Could you check a few things on this model? Use its own coordinates, in mm. A direction names the side the tool comes from. Give positions to 0.01 mm unless a question says otherwise; leave off trailing zeros. Loops run counter-clockwise (first coordinate to the right, second up) from the corner with the lowest first, then second, coordinate; pieces in that order, holes last. Notation, with made-up numbers: M -35,12.5 L -30,12.5 A17 cw -30,37.5 Z; hole C -17.5,3 d7. An arc over 180 degrees is marked long. Use a Markdown table: item, result. Add a question column.
1) Suppose I cut it at D-D on y = 71. List the corners of the cut face in (x, z) for me, and give its area (3 significant figures).
2) If I drill on line 1 along Y through (x, z) = (2.5, -18.5); line 2 along X through (y, z) = (62, 0); line 3 along Z through (x, y) = (0, 62.5), over which ranges is the centre line in solid material (lowest first)? Write a range as [from, to].
3) Will these pins go through, and if not, where does the flat tip stop? pin 1 Ø4 at (y, z) = (63, -25.5) entering from -X; pin 2 Ø17.5 at (y, z) = (44.5, -14.5) entering from -X; pin 3 Ø10 at (x, z) = (-4.5, -27) entering from +Y.
4) We'd pull the mould along Y, two halves only. Please class faces 6 (the flat face through (6, 65, -23)), 7 (the cylindrical face through (1.14, 31.85, 19.25)), 8 (the flat face through (0, 0, -9)), 9 (the flat face through (-13, 50, 0)): +Y half, -Y half, draft (parallel to the pull), parting line (faces both ways), or undercut.
5) Suppose I cut it at C-C on z = 0. List the corners of the cut face in (x, y) for me.
6) Suppose I cut it at B-B on y = 34.5. List the corners of the cut face in (x, z) for me, and give its area (3 significant figures).
7) Suppose I cut it at A-A on z = -16.5. List the corners of the cut face in (x, y) for me.
8) Which directions (+Z, -Z, +X, -X, +Y, -Y) give clear straight access to the entire face, cutting with the end or side of a thin tool? Please do faces 1 (the cylindrical face through (5, 65, -34)), 2 (the flat face through (11.774, 62.762, 8.74)), 3 (the flat face through (-1, 80, 13)), 4 (the cylindrical face through (-7.835, 64.345, 9.739)), 5 (the cylindrical face through (0.15, 48.33, 13.25)).
```python
from build123d import *
from OCP.BRepFilletAPI import BRepFilletAPI_MakeFillet

# Parameters (mm, degrees)
SKETCH1_R               = 12.5
BOSS_EXTRUDE1_DEPTH     = 80
CUT_EXTRUDE1_DEPTH      = 88.77439656
CUT_EXTRUDE1_DEPTH_BACK = 88.77439656
SKETCH4_OUTSIDE_W       = 61.818
SKETCH4_OUTSIDE_H       = 100.83
SKETCH6_W               = 20
SKETCH6_H               = 8.19180338
SKETCH6_W_2             = 12
SKETCH6_H_2             = 19
BOSS_EXTRUDE3_DEPTH     = 50
CUT_EXTRUDE2_START      = -30
SKETCH8_R               = 12.5
CUT_EXTRUDE2_DEPTH      = 30
FILLET1_R               = 5
FILLET2_R               = 15
FILLET3_R1              = 1
FILLET3_R2              = 5
CUT_EXTRUDE4_DEPTH      = 84.91706908
CUT_EXTRUDE4_DEPTH_BACK = 84.91706908
SKETCH11_R              = 1.55
FILLET4_R               = 10
SKETCH12_R              = 5.25
CUT_EXTRUDE5_DEPTH      = 96.372952239


with BuildPart() as part:
    # Sketch1 → Boss-Extrude1 (new body)
    with BuildSketch(Plane(origin=(0, 0, 0), x_dir=(1, 0, 0), z_dir=(0, 1, 0))):
        with BuildLine():
            Line((-13.243243243, -4.540540541), (-10, -14))
            Line((-10, -14), (-10, -26.98786193))
            Line((-10, -26.98786193), (10, -26.98786193))
            Line((10, -26.98786193), (10, -14))
            Line((10, -14), (13.597983435, -3.330892747))
            ThreePointArc((13.597983435, -3.330892747), (-0.630295246, 13.985804514), (-13.243243243, -4.540540541))
        make_face()
        with Locations(Location((0, 0, 0), (0, 0, 270))):
            Circle(SKETCH1_R, mode=Mode.SUBTRACT)
    extrude(amount=BOSS_EXTRUDE1_DEPTH)

    # Sketch4 outside → Cut-Extrude1 (cut, two sides: drawn at the far end of the back side and taken through both)
    with BuildSketch(Plane.ZY.offset(10).offset(-CUT_EXTRUDE1_DEPTH_BACK)):
        with Locations((6.494, 40)):
            Rectangle(SKETCH4_OUTSIDE_W, SKETCH4_OUTSIDE_H)
        with BuildLine():
            Line((-10, 50), (10, 50))
            ThreePointArc((10, 50), (12.828427125, 48.828427125), (14, 46))
            Line((14, 46), (14, 0))
            Line((14, 0), (23.289589956, 0))
            ThreePointArc((23.289589956, 0), (26.209542913, 8.210116535), (25.999737715, 16.921495334))
            Line((25.999737715, 16.921495334), (19.944041303, 78.646458452))
            ThreePointArc((19.944041303, 78.646458452), (19.458758034, 79.611235276), (18.451208451, 80))
            Line((18.451208451, 80), (14, 80))
            Line((14, 80), (-10, 80))
            ThreePointArc((-10, 80), (-12.828427125, 78.828427125), (-14, 76))
            Line((-14, 76), (-14, 54))
            ThreePointArc((-14, 54), (-12.828427125, 51.171572875), (-10, 50))
        make_face(mode=Mode.SUBTRACT)
    extrude(amount=CUT_EXTRUDE1_DEPTH + CUT_EXTRUDE1_DEPTH_BACK, mode=Mode.SUBTRACT)

    # Sketch6 → Boss-Extrude3 (add)
    with BuildSketch(Plane(origin=(0, 0, 14), x_dir=(-1, 0, 0), z_dir=(0, 0, -1))):
        with Locations((0, 4.09590169)):
            Rectangle(SKETCH6_W, SKETCH6_H)
        with Locations((0, 64.998822006)):
            Rectangle(SKETCH6_W_2, SKETCH6_H_2)
    extrude(amount=BOSS_EXTRUDE3_DEPTH)

    # Sketch8 → Cut-Extrude2 (cut)
    with BuildSketch(Plane(origin=(0, 80, 0), x_dir=(1, 0, 0), z_dir=(0, 1, 0)).offset(CUT_EXTRUDE2_START)):
        with Locations(Location((0, 0, 0), (0, 0, 53.130102354))):
            Circle(SKETCH8_R)
    extrude(amount=CUT_EXTRUDE2_DEPTH, mode=Mode.SUBTRACT)

    # Fillet1
    fillet1_edges = [part.edges().sort_by_distance(p)[0] for p in [
        (10, 4.09590169, -36),
        (-10, 4.09590169, -36),
        (6, 64.998822006, -36),
        (-6, 64.998822006, -36),
    ]]
    fillet(fillet1_edges, radius=FILLET1_R)

    # Fillet2
    fillet2_edges = [part.edges().sort_by_distance(p)[0] for p in [
        (0, 8.19180338, 14),
    ]]
    fillet(fillet2_edges, radius=FILLET2_R)

    # Fillet3: one fillet with a radius per group of edges: ONE call of the kernel's fillet builder (fillet() takes one radius for all edges)
    fillet3_edges_1 = [part.edges().sort_by_distance(p)[0] for p in [
        (0, 74.498822006, -14),
        (0, 55.498822006, -14),
    ]]
    fillet3_edges_2 = [part.edges().sort_by_distance(p)[0] for p in [
        (-6, 64.998822006, -12.649110641),
        (6, 64.998822006, -12.649110641),
    ]]
    fillet3 = BRepFilletAPI_MakeFillet(part.part.solid().wrapped)
    for e in fillet3_edges_1:
        fillet3.Add(FILLET3_R1, e.wrapped)
    for e in fillet3_edges_2:
        fillet3.Add(FILLET3_R2, e.wrapped)
    add(Compound.cast(fillet3.Shape()), mode=Mode.REPLACE)

    # Sketch11 → Cut-Extrude4 (cut, two sides: drawn at the far end of the back side and taken through both)
    with BuildSketch(Plane(origin=(0, 74.498822006, 0), x_dir=(1, 0, 0), z_dir=(0, 1, 0)).offset(-CUT_EXTRUDE4_DEPTH_BACK)):
        with Locations(Location((0, 31.585251235, 0), (0, 0, 270))):
            Circle(SKETCH11_R)
    extrude(amount=CUT_EXTRUDE4_DEPTH + CUT_EXTRUDE4_DEPTH_BACK, mode=Mode.SUBTRACT)

    # Fillet4
    fillet4_edges = [part.edges().sort_by_distance(p)[0] for p in [
        (0, 16.921495334, 25.999737715),
        (0, 0, 23.289589956),
    ]]
    fillet(fillet4_edges, radius=FILLET4_R)

    # Sketch12 → Cut-Extrude5 (cut, through all)
    with BuildSketch(Plane(origin=(0, 0, 14), x_dir=(-1, 0, 0), z_dir=(0, 0, -1))):
        with Locations((0, 36.973808643)):
            Circle(SKETCH12_R)
    extrude(amount=-CUT_EXTRUDE5_DEPTH, mode=Mode.SUBTRACT)


solid = part.part
```
Answer block:
| question | item | result |
|---|---|---|
| 1 | outline | M -13.24,4.54 A14 ccw -8.11,-11.42 A5 cw -6,-15.49 L -6,-31 A5 ccw -1,-36 L 1,-36 A5 ccw 6,-31 L 6,-15.49 A5 cw 8.11,-11.42 A14 ccw 13.6,3.33 L 10,14 L 10,20.69 L -10,20.69 L -10,14 Z; hole C 0,0 d25; hole C 0,-31.59 d3.1 |
| 1 | area | 549 mm^2 |
| 2 | line 1 | y = [0, 8.19], [55.5, 74.5] |
| 2 | line 2 | x = [-14, -12.5], [12.5, 14] |
| 2 | line 3 | z = [-36, -33.14], [-30.04, -12.5], [12.5, 21.53] |
| 3 | pin 1 | stops at x = -6 |
| 3 | pin 2 | stops at x = -11.7 |
| 3 | pin 3 | stops at y = 74.5 |
| 4 | face 6 | draft |
| 4 | face 7 | undercut |
| 4 | face 8 | -Y half |
| 4 | face 9 | undercut |
| 5 | outline | M -14,50 L -12.5,50 L -12.5,80 L -14,80 Z; M -10,0 L 10,0 L 10,8.23 L -10,8.23 Z; M 12.5,50 L 14,50 L 14,80 L 12.5,80 Z |
| 6 | outline | M -10,14 L -4.63,14 L -4.63,24.28 L -10,24.28 Z; M 4.63,14 L 10,14 L 10,24.28 L 4.63,24.28 Z |
| 6 | area | 110 mm^2 |
| 7 | outline | M -10,0 L 10,0 L 10,8.19 L -10,8.19 Z; M -6,55.5 L 6,55.5 L 6,74.5 L -6,74.5 Z |
| 8 | face 1 | -Z, +X, +Y |
| 8 | face 2 | +Z, +X, +Y, -Y |
| 8 | face 3 | +Z, -Z, +X, -X, +Y |
| 8 | face 4 | +Y |
| 8 | face 5 | -Z, +X, -X |
